Input: part model. Units: mm. Frame: model coordinates. A direction names the side the tool comes from. Give positions to 0.01 mm unless a question says otherwise; leave off trailing zeros. Loops run counter-clockwise (first coordinate to the right, second up) from the corner with the lowest first, then second, coordinate; pieces in that order, holes last. Notation, with made-up numbers: (-4, 49) - (42, 49) arc R18 cw to (42, 78) - close; hole circle Ø1 at (-36, 13). An arc over 180 degrees is marked (long way). Answer as a JSON object with one key per item and string values. Group by question number.
(1) Section query A-A (z = 4.5). Return loops of the section in (x, y), plus the area to 3 significant figures.
(2) Mould query, pull axis Y, two halves, no side actions, for faces 4 (the flat face through (0, 1, 1)), 5 (the cylindrical face through (-1.5, 0.07, 10.51)), 6 (the flat face through (0, 0, 19)). Classes: +Y half, -Y half, draft (parallel to the pull), parting line (faces both ways), or undercut.
(3) Material intervals for L1, parallel to Z at x = 0.25, y = 0.85; L2, parallel to Y at x = -1, z = 4.25; L3, parallel to Z at x = -1.45, y = -2, sorted ascending.
(4) Access query for faces 1 (the cylindrical face through (-0.596, -2.685, 1.549)), 2 (the flat face through (0, 0, 1.5)), 3 (the flat face through (1, 2, 2)). Directions: +Z, -Z, +X, -X, +Y, -Y. A direction counts if a zero-diameter tool reaches every point of the face in a straight line with its end or side. Return the directions, or none.
(5) Pin query (flat end, axial travel): P1, Ø2, axis at y = -0.5, z = 14, coming from the -X side; P2, Ø3, axis at x = -2, z = 9.5, coming from the +Y side; P3, Ø1.5, axis at x = 0, z = 17, coming from the -Y side. Return the tip coordinate at first contact, or that it passes through.
```python
from build123d import *

# Parameters (mm, degrees)
F1_R     = 2.75
F1_R_2   = 1.5
F2_DEPTH = 2
F3_START = 1.5
F3_DEPTH = 0.5
F4_START = 2
F4_DEPTH = 17
F5_SIZE2 = 1.25
F5_SIZE  = 1.25
F6_R     = 0.25


# Not quite as in the source:
# - a feature names something its author has since deleted; it is built from what else it names


with BuildPart() as f2:
    # F1 (on Top) → F2 (new body)
    with BuildSketch(Plane.XY):
        Circle(F1_R)
        Circle(F1_R_2, mode=Mode.SUBTRACT)
        Circle(F1_R_2)
        Polygon((-0.5773502692, -1), (-1.1547005384, 0), (-0.5773502692, 1), (0.5773502692, 1), (1.1547005384, 0), (0.5773502692, -1), align=None, mode=Mode.SUBTRACT)
    extrude(amount=F2_DEPTH)

    # F1 (on Top) → F3 (join)
    with BuildSketch(Plane.XY.offset(F3_START)):
        Polygon((-0.5773502692, 1), (-1.1547005384, 0), (-0.5773502692, -1), (0.5773502692, -1), (1.1547005384, 0), (0.5773502692, 1), align=None)
    extrude(amount=F3_DEPTH)

    # F1 (on Top) → F4 (join)
    with BuildSketch(Plane.XY.offset(F4_START)):
        Circle(F1_R_2)
        Polygon((-0.5773502692, -1), (-1.1547005384, 0), (-0.5773502692, 1), (0.5773502692, 1), (1.1547005384, 0), (0.5773502692, -1), align=None, mode=Mode.SUBTRACT)
        Polygon((-0.5773502692, 1), (-1.1547005384, 0), (-0.5773502692, -1), (0.5773502692, -1), (1.1547005384, 0), (0.5773502692, 1), align=None)
    extrude(amount=F4_DEPTH)

    # F5
    f5_edges = [f2.edges().sort_by_distance(p)[0] for p in [
        (-2.75, 0, 0),
    ]]
    chamfer(f5_edges, length=F5_SIZE, length2=F5_SIZE2)

    # F6
    f6_edges = [f2.edges().sort_by_distance(p)[0] for p in [
        (-2.75, 0, 2),
        (-1.5, 0, 2),
        (-1.5, 0, 0),
        (-2.75, 0, 1.25),
    ]]
    fillet(f6_edges, radius=F6_R)


solid = f2.part
```
Recorded:
{
 "1": {"outline": "circle Ø3 at (0, 0)", "area": "7.07 mm^2"},
 "2": {"face 4": "undercut", "face 5": "parting line", "face 6": "draft"},
 "3": {"L1": "z = 1.5 to 19", "L2": "y = -1.12 to 1.12", "L3": "z = 0.97 to 2"},
 "4": {"face 1": "+Z, -Z", "face 2": "-Z", "face 3": "+Z"},
 "5": {"P1": "stops at x = -1.5", "P2": "stops at y = 1.41", "P3": "stops at y = -1.5"}
}
